For this review, use the dimensioned drawing (mm, ordinates from the lowest corner) and the shaded views. A direction names the side the tool comes from. Give positions to 0.01 mm unless a question says otherwise; leave off trailing zeros. Loops run counter-clockwise (first coordinate to the right, second up) from the corner with the lowest first, then second, coordinate; pieces in that order, holes last. Notation, with made-up numbers: M 43,23 L 52,23 A17 ccw 52,41 Z; hole C 25.25,-25.5 d11. An arc over 180 degrees is marked long. Use CSV: the item, a comma, the result in double quotes.
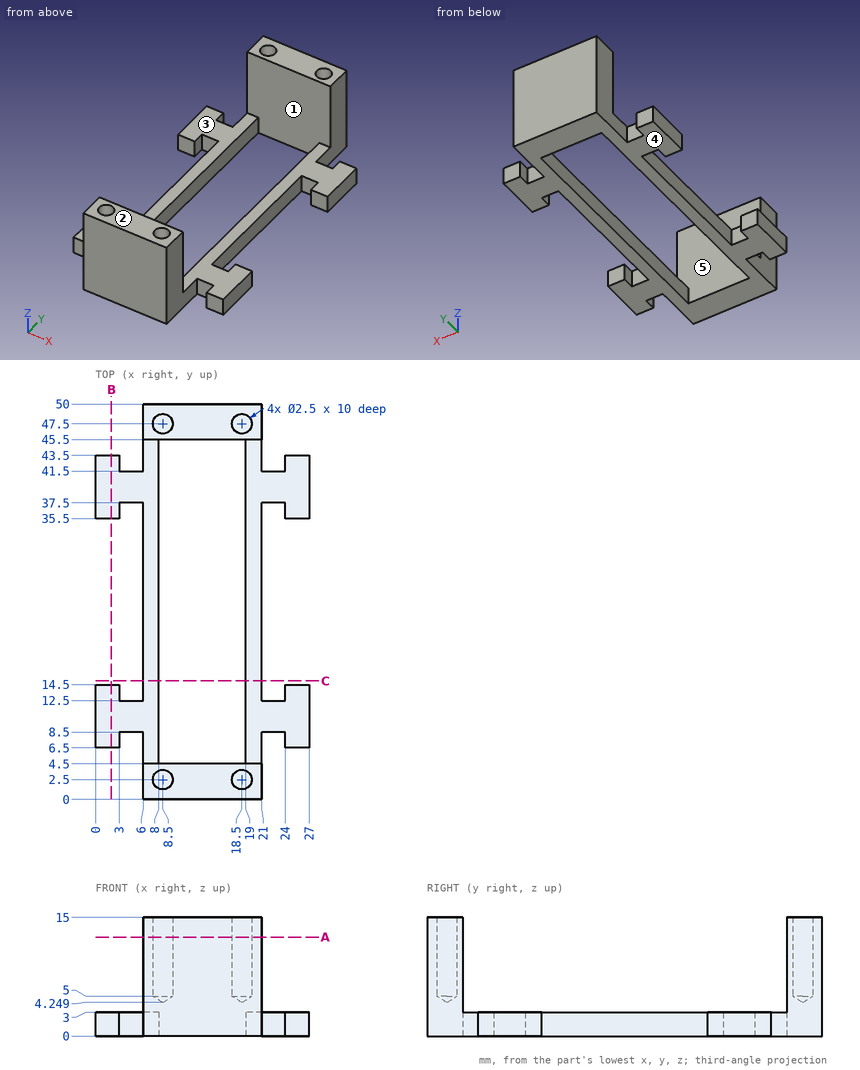
(1) We need section C-C on y = 15. State the section outline as (x, z) points, then the cut area to 3 significant figures.
A:
outline,"M 6,0 L 8,0 L 8,3 L 6,3 Z; M 19,0 L 21,0 L 21,3 L 19,3 Z"
area,"12.0 mm²"
(2) Machinability: for the marked faces 3, 4 and 5, which of the approach directions +Z, -Z, +X, -X, +Y, -Y give a long, thin tool a straight path to every point of the face, cutting with its end or side? Answer none if there is none.
A:
face 3,"+Z, +X, -X"
face 4,"-Z, +X, -X, +Y, -Y"
face 5,"+Z"
(3) We need section A-A on z = 12.5. State the section outline as (x, y) points, then the cut area to 3 significant figures.
A:
outline,"M 6,0 L 21,0 L 21,4.5 L 6,4.5 Z; M 6,45.5 L 21,45.5 L 21,50 L 6,50 Z; hole C 8.5,2.5 d2.5; hole C 8.5,47.5 d2.5; hole C 18.5,2.5 d2.5; hole C 18.5,47.5 d2.5"
area,"115 mm²"
(4) We need section B-B on x = 2. State the section outline as (y, z) points.
A:
outline,"M 6.5,0 L 14.5,0 L 14.5,3 L 6.5,3 Z; M 35.5,0 L 43.5,0 L 43.5,3 L 35.5,3 Z"
(5) Wall thickness on line 1 along X through (y, z) = (47.5, 10); line 2 along Y through (x, z) = (8.5, 7); line 3 along Y through (x, z) = (19.5, 13.75): over which ranges is each line inside the solid? List them lowest first. Write a range as [from, to].
A:
line 1,"[6, 7.25], [9.75, 17.25], [19.75, 21]"
line 2,"[0, 1.25], [3.75, 4.5], [45.5, 46.25], [48.75, 50]"
line 3,"[0, 1.75], [3.25, 4.5], [45.5, 46.75], [48.25, 50]"
(6) Clearance check with flat-ended pins moving along their axes: P1, Ø3, axis at x = 8.5, y = 2.5, coming from the -Z side; P2, Ø1.5, axis at x = 25, z = 1.5, coming from the +Y side; P3, Ø4, axis at y = 47.5, z = 5.5, coming from the +X side; P4, Ø2.5, axis at x = 22, y = 16.5, coming from the +Z side. State where each tip first meets the part, or that it passes through.
A:
P1,"z = 0"
P2,"y = 43.5"
P3,"x = 21"
P4,"z = 3"
(7) The part is to be moulded in two halves that separate along X. For the marked faces 1 and 2, say which applies: released by +X, released by -X, zero draft, split by the parting line, or undercut.
A:
face 1,"undercut"
face 2,"zero draft"
